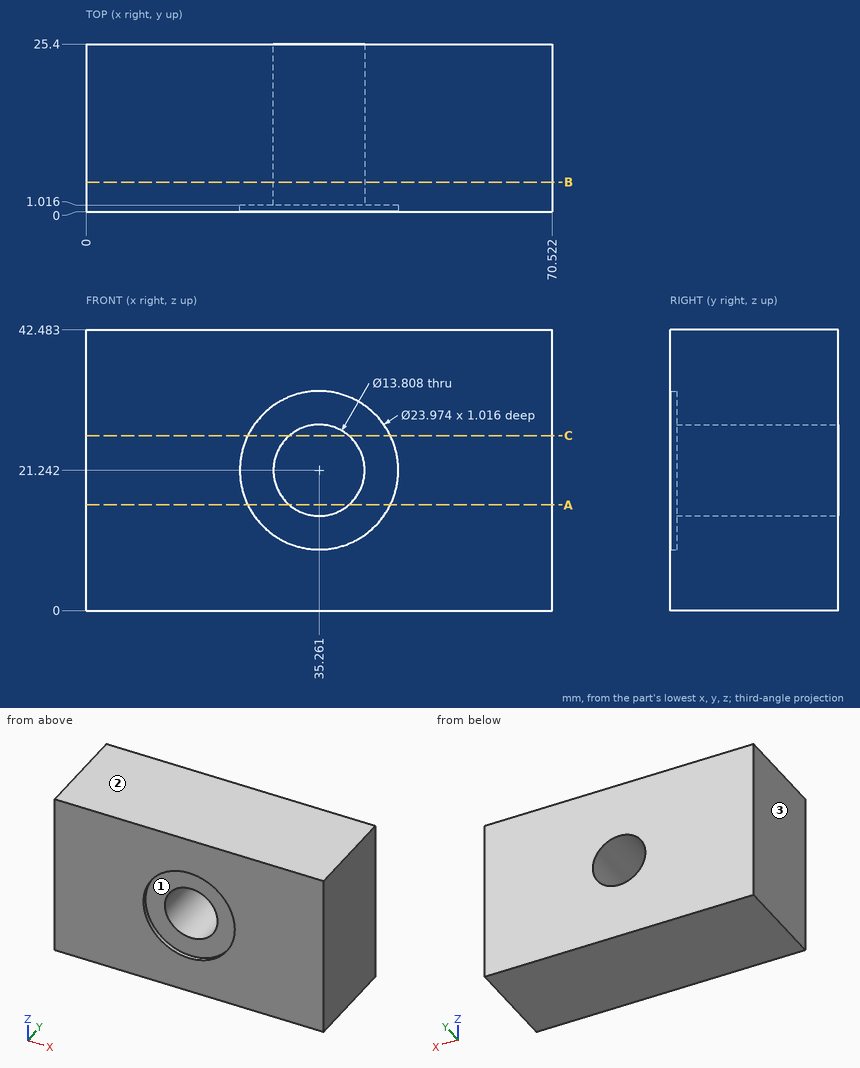
Job drawing, mm, ordinate dimensions from the low corner. One solid piece. Round coordinates to 2 decimals unless told otherwise and drop trailing zeros. Loops run counter-clockwise (first coordinate to the right, second up) from the corner with the lowest first, then second, coordinate; pieces in that order, holes last.
Item 1: Cut at A-A, the plane z = 16. Give the cut face in (x, y) (1 decimal), then the cut area to 3 significant figures.
Item 2: Mould opens along Z. For the marked faces 1, 2 and 3 say: +Z half, -Z half, draft (parallel to the pull), parting line (faces both ways), or undercut.
Item 3: Drop flat-ended pins along their axis: P1, Ø5, axis at x = 35, y = 23, coming from the -Z side; P2, Ø16, axis at x = 35.26, z = 21.24, coming from the -Y side. Give the stop position or say it passes through.
Item 4: Cut at C-C, the plane z = 26.5. Give the cut face in (x, y) (1 decimal), then the cut area to 3 significant figures.
Item 5: Drill centre lines: line 1 (X direction, y = 19, z = 24); line 2 (X direction, y = 5.5, z = 15) (1 decimal); line 3 (Z direction, x = 34.5, y = 11). Where is each one in solid material? Low to high.
Item 6: Cut at B-B, the plane y = 4.5. Give the cut face in (x, z) (1 decimal), then the cut area to 3 significant figures.
A:
1. outline: (0, 0) - (24.5, 0) - (24.5, 1) - (30.8, 1) - (30.8, 25.4) - (0, 25.4) - close; (39.8, 1) - (46, 1) - (46, 0) - (70.5, 0) - (70.5, 25.4) - (39.8, 25.4) - close
1. area: 1,550 mm2
2. face 1: undercut
2. face 2: +Z half
2. face 3: draft
3. P1: stops at z = 0
3. P2: stops at y = 1.02
4. outline: (0, 0) - (24.5, 0) - (24.5, 1) - (30.8, 1) - (30.8, 25.4) - (0, 25.4) - close; (39.7, 1) - (46, 1) - (46, 0) - (70.5, 0) - (70.5, 25.4) - (39.7, 25.4) - close
4. area: 1,550 mm2
5. line 1: x = 0 to 28.93, 41.59 to 70.52
5. line 2: x = 0 to 32.3, 38.2 to 70.5
5. line 3: z = 0 to 14.38, 28.1 to 42.48
6. outline: (0, 0) - (70.5, 0) - (70.5, 42.5) - (0, 42.5) - close; hole circle Ø13.8 at (35.3, 21.2)
6. area: 2,850 mm2
